```python
from build123d import *

# Parameters (mm, degrees)
SKETCH2_W           = 50.8
SKETCH2_H           = 25.4
SKETCH2_W_2         = 45.72
SKETCH2_H_2         = 20.32
BOSS_EXTRUDE1_DEPTH = 711.2
SKETCH3_R           = 2.54
CUT_EXTRUDE1_DEPTH  = 51.8
LPATTERN1_COUNT     = 28
LPATTERN1_PITCH     = 25.4


with BuildPart() as part:
    # Sketch2 → Boss-Extrude1 (new body)
    with BuildSketch(Plane(origin=(0, 0, 0), x_dir=(0, 0, -1), z_dir=(1, 0, 0))):
        with Locations((25.4, 12.7)):
            Rectangle(SKETCH2_W, SKETCH2_H)
        with Locations((25.4, 12.7)):
            Rectangle(SKETCH2_W_2, SKETCH2_H_2, mode=Mode.SUBTRACT)
    extrude(amount=BOSS_EXTRUDE1_DEPTH)

    # Sketch3 → Cut-Extrude1 (cut, through all)
    with BuildSketch(Plane.XY):
        with Locations((12.7, 12.7)):
            Circle(SKETCH3_R)
    cut_extrude1 = extrude(amount=-CUT_EXTRUDE1_DEPTH, mode=Mode.SUBTRACT)

    # LPattern1: Cut-Extrude1 ×28
    with Locations(*[(i * LPATTERN1_PITCH, 0, 0) for i in range(1, LPATTERN1_COUNT)]):
        add(cut_extrude1, mode=Mode.SUBTRACT)


solid = part.part
```
The listing builds one solid part. Answer for the finished solid, in the listing's coordinates (mm). A direction names the side the tool comes from. Coordinates: 2 decimals unless noted, no trailing zeros. Loops run counter-clockwise (first coordinate to the right, second up) from the corner with the lowest first, then second, coordinate; pieces in that order, holes last. Notation, with made-up numbers: (-15.75, 75) - (-4.75, 75) arc R24 ccw to (-4.75, 94) - close; hole circle Ø10 at (-1.5, -40). An arc over 180 degrees is marked (long way). Use a Markdown table: item, result. Add a question column.
1) The part is cut by section A-A, the plane z = -34.5. Give the vertices of the cut face in (x, y).
2) The part is cut by section B-B, the plane x = 478.5. Give the vertices of the cut face in (y, z).
3) For faces 1 (the flat face through (351, 22.86, -25)), 2 (the flat face through (0, 2, -23)), determine the directions among +Z, -Z, +X, -X, +Y, -Y from which every point of the face is accessible in a straight line to the end or side of a thin tool.
4) Find the intervals of material crossed by line 1 (Y direction, x = 337, z = -37); line 2 (Z direction, x = 681, y = 20); line 3 (Y direction, x = 419.1, z = -2), in increasing order.
5) The mould has two halves that part along Z. Classify faces 3 (the flat face through (351, 13, 0)), 4 (the flat face through (351, 0, -25)), 5 (the flat face through (351, 13, -48.26)), 6 (the flat face through (351, 13, -50.8)): released by +Z, released by -Z, zero draft, split by the parting line, or undercut.
6) Given pin 1 (8 mm diameter, centred on x = 520.7, y = 12.7, fed in from -Z); pin 2 (4.5 mm diameter, centred on x = 444.5, y = 12.7, fed in from -Z), each flat-ended and moving along its own axis, determine where each tip first touches the part or whether it passes through.
Here are the results:
| question | item | result |
|---|---|---|
| 1 | outline | (0, 0) - (711.2, 0) - (711.2, 2.54) - (0, 2.54) - close; (0, 22.86) - (711.2, 22.86) - (711.2, 25.4) - (0, 25.4) - close |
| 2 | outline | (0, -50.8) - (25.4, -50.8) - (25.4, 0) - (0, 0) - close; hole (2.54, -48.26) - (22.86, -48.26) - (22.86, -2.54) - (2.54, -2.54) - close |
| 3 | face 1 | +X, -X |
| 3 | face 2 | +Z, -Z, -X, +Y, -Y |
| 4 | line 1 | y = 0 to 2.54, 22.86 to 25.4 |
| 4 | line 2 | z = -50.8 to -48.26, -2.54 to 0 |
| 4 | line 3 | y = 0 to 10.16, 15.24 to 25.4 |
| 5 | face 3 | released by +Z |
| 5 | face 4 | zero draft |
| 5 | face 5 | undercut |
| 5 | face 6 | released by -Z |
| 6 | pin 1 | stops at z = -50.8 |
| 6 | pin 2 | passes through |
